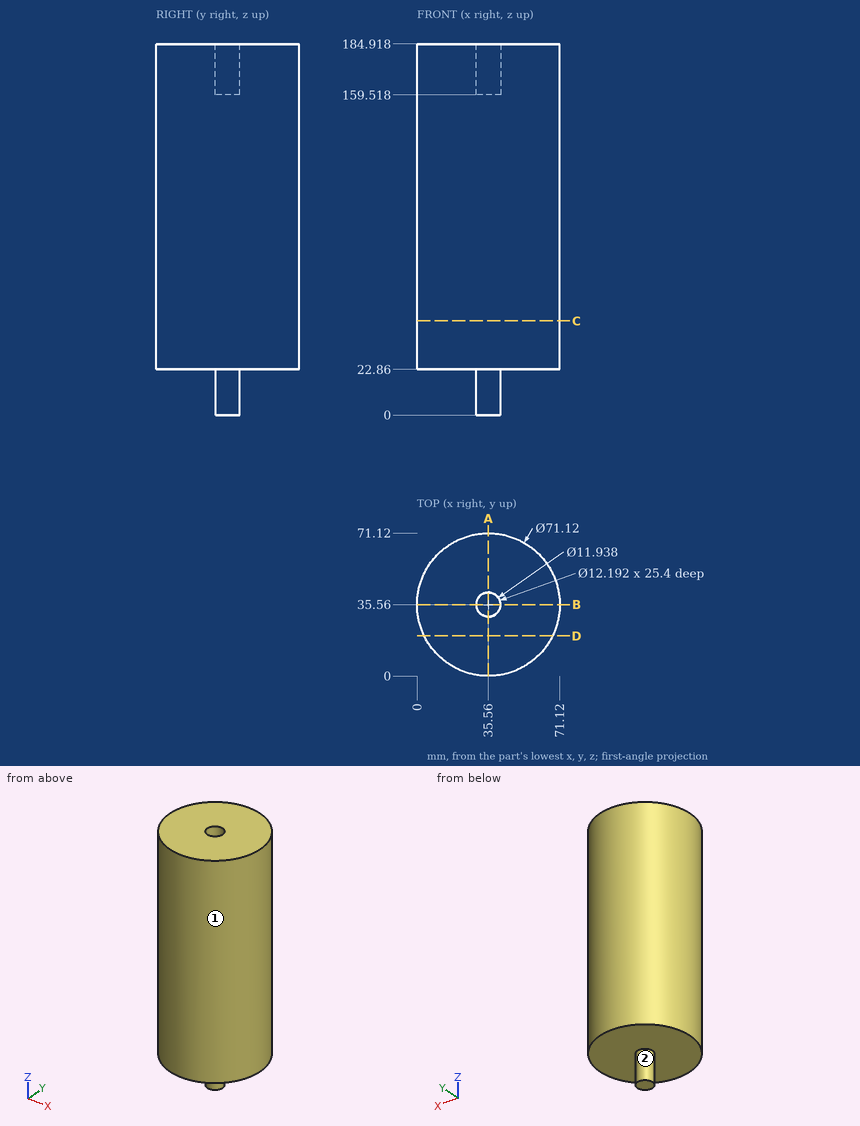
Here's the drawing with two shaded views (mm, measured from the low corner). I have some questions. A direction names the side the tool comes from. Give positions to 0.01 mm unless a question says otherwise; leave off trailing zeros. Loops run counter-clockwise (first coordinate to the right, second up) from the corner with the lowest first, then second, coordinate; pieces in that order, holes last. Notation, with made-up numbers: M 10.25,-5 L 48.25,-5 A10 cw 48.25,4 Z; hole C 69.25,87.25 d10. An arc over 180 degrees is marked long. Use one line per item in the form item = value. Start each with the question number.
(1) I want a section at A-A, the plane x = 35.56. Write out the boundary of the cut face in (y, z), and give its area (3 significant figures).
(2) On a 3-axis mill with a long thin cutter (end or side, diameter ignored), from which of +Z, -Z, +X, -X, +Y, -Y can I reach the whole of each face in a straight line? I mean the marked faces 1 and 2. Say none if no direction works.
(3) I'm going to push flat-ended pins straight in: P1, Ø5, axis at y = 12.5, z = 33.5, coming from the +X side; P2, Ø4, axis at x = 35, y = 57, coming from the -Z side; P3, Ø8, axis at y = 40, z = 139.5, coming from the +X side. Where does each tip first touch, or does it pass through?
(4) Please list where these lines run through material, in increasing order: line 1 (Y direction, x = 35, z = 166) (1 decimal); line 2 (Y direction, x = 35.56, z = 172.5); line 3 (Z direction, x = 46, y = 47).
(5) I want a section at C-C, the plane z = 47. Write out the boundary of the cut face in (x, y).
(6) I want a section at D-D, the plane y = 20. Write out the boundary of the cut face in (x, z) (1 decimal).
Worked out:
q1.outline = M 0,22.86 L 29.59,22.86 L 29.59,0 L 41.53,0 L 41.53,22.86 L 71.12,22.86 L 71.12,184.92 L 41.66,184.92 L 41.66,159.52 L 29.46,159.52 L 29.46,184.92 L 0,184.92 Z
q1.area = 11,500 mm²
q2.face_1 = +Z, -Z
q2.face_2 = -Z
q3.P1 = 64.57
q3.P2 = 22.86
q3.P3 = 71.12
q4.line_1 = 0 to 29.5, 41.6 to 71.1
q4.line_2 = 0 to 29.46, 41.66 to 71.12
q4.line_3 = 22.86 to 184.92
q5.outline = C 35.56,35.56 d71.12
q6.outline = M 3.6,22.9 L 67.5,22.9 L 67.5,184.9 L 3.6,184.9 Z
